Verification items for the finished model (mm, model axes). Face numbers are marked on the shaded views. Round coordinates to 2 decimals unless told otherwise and drop trailing zeros. Write each loop counter-clockwise with the first axis right and the second up, starting at its lowest first coordinate (ties: lowest second). Pieces come first, ordered by that corner, then holes. Notation, with made-up numbers: (-12, 28) - (23, 28) arc R16 ccw to (23, 38) - close; hole circle Ø10 at (61.25, 42). An arc over 180 degrees is marked (long way). Answer as a JSON object with one key per item and string values.
```python
from build123d import *

# Parameters (mm, degrees)
SKETCH1_R           = 25.5
SKETCH1_R_2         = 8.5
BOSS_EXTRUDE1_DEPTH = 5
CIRPATTERN1_COUNT   = 6


with BuildPart() as part:
    # Sketch1 → Boss-Extrude1 (new body)
    with BuildSketch(Plane.XY):
        Circle(SKETCH1_R)
        Circle(SKETCH1_R_2, mode=Mode.SUBTRACT)
    extrude(amount=BOSS_EXTRUDE1_DEPTH)

    # Sketch3 → M3 Clearance Hole1 (revolve, cut)
    with BuildSketch(Plane(origin=(0, 22.5, 5), x_dir=(0, -1, 0), z_dir=(1, 0, 0))):
        Polygon((0, 0), (0, 11.021463052), (1.7, 10), (1.7, 0), align=None)
    m3_clearance_hole1 = revolve(axis=Axis((0, 22.5, 11.35), (0, 0, -1)), mode=Mode.SUBTRACT)

    # Sketch5 → CSK for M3 Countersunk Flat Head Screw3 (revolve, cut)
    with BuildSketch(Plane(origin=(0, 11.5, 5), x_dir=(0, -1, 0), z_dir=(1, 0, 0))):
        Polygon((0, 0), (0, 11.021463052), (1.7, 10), (1.7, 1.45), (3.15, 0), align=None)
    csk_for_m3_countersunk_flat_head_screw3 = revolve(axis=Axis((0, 11.5, 11.35), (0, 0, -1)), mode=Mode.SUBTRACT)

    # CirPattern1: M3 Clearance Hole1, CSK for M3 Countersunk Flat Head Screw3 ×6 about axis
    cirpattern1_axis = Axis((0, 0, 0), (0, 0, 1))
    for i in range(1, CIRPATTERN1_COUNT):
        add(m3_clearance_hole1.rotate(cirpattern1_axis, i * 360 / CIRPATTERN1_COUNT), mode=Mode.SUBTRACT)
        add(csk_for_m3_countersunk_flat_head_screw3.rotate(cirpattern1_axis, i * 360 / CIRPATTERN1_COUNT), mode=Mode.SUBTRACT)


solid = part.part
```
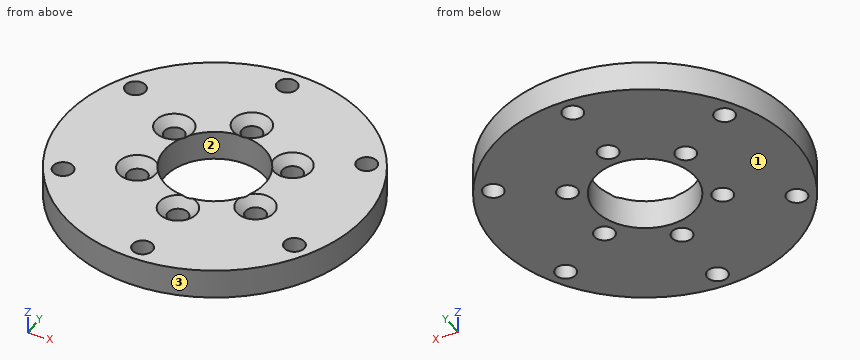
Q1. Material ranges on line 1 along Y through (x, z) = (0, 2.45); line 2 along X through (y, z) = (-7, 1.05); line 3 along Y through (x, z) = (20.5, 4.3), recorded low to high. Write a range as [from, to].
Geometry check:
{"line 1": "y = [-25.5, -24.2], [-20.8, -13.2], [-9.8, -8.5], [8.5, 9.8], [13.2, 20.8], [24.2, 25.5]", "line 2": "x = [-24.52, -11.11], [-8.81, -4.82], [4.82, 8.81], [11.11, 24.52]", "line 3": "y = [-15.17, -12.61], [-9.89, 9.89], [12.61, 15.17]"}
Q2. Gauge pin test, flat ends, axial feed: P1, Ø3, axis at x = -9.96, y = 5.75, coming from the +Z side; P2, Ø1.5, axis at x = -18.5, z = 2, coming from the +Y side; P3, Ø4, axis at x = -9.96, y = -5.75, coming from the +Z side; P4, Ø1, axis at x = 5, z = 2, coming from the -Y side. Record the tip position at first contact, or that the pin passes through.
Geometry check:
{"P1": "passes through", "P2": "stops at y = 18.31", "P3": "stops at z = 3.85", "P4": "stops at y = -25.1"}
Q3. Section check D-D, the plane y = -11.5. Record the cut outline in (x, z).
Geometry check:
{"outline": "(-22.76, 0) - (-21.17, 0) - (-21.17, 5) - (-22.76, 5) - close; (-17.8, 0) - (-1.7, 0) - (-1.7, 3.55) - (-3.15, 5) - (-17.8, 5) - close; (1.7, 0) - (17.8, 0) - (17.8, 5) - (3.15, 5) - (1.7, 3.55) - close; (21.17, 0) - (22.76, 0) - (22.76, 5) - (21.17, 5) - close"}
Q4. Section check C-C, the plane z = 0.9. State how many separate pieces and enclosed holes the cut face has, then the cut area to 3 significant figures.
Geometry check:
{"separate pieces": "1", "enclosed holes": "13", "area": "1,710 mm2"}
Q5. Section check A-A, the plane y = 22.5. Record the cut outline in (x, z).
Geometry check:
{"outline": "(-12, 0) - (-1.7, 0) - (-1.7, 5) - (-12, 5) - close; (1.7, 0) - (12, 0) - (12, 5) - (1.7, 5) - close"}
Q6. Release check for a two-part mould opening along Y. For the marked faces 1, 2 and 3 record: released by +Y, released by -Y, zero draft, split by the parting line, or undercut.
Geometry check:
{"face 1": "zero draft", "face 2": "undercut", "face 3": "split by the parting line"}
Q7. Section check B-B, the plane x = 0. Record the cut outline in (y, z), then the cut area to 3 significant figures.
Geometry check:
{"outline": "(-25.5, 0) - (-24.2, 0) - (-24.2, 5) - (-25.5, 5) - close; (-20.8, 0) - (-13.2, 0) - (-13.2, 3.55) - (-14.65, 5) - (-20.8, 5) - close; (-9.8, 0) - (-8.5, 0) - (-8.5, 4.85) - (-9.8, 3.55) - close; (8.5, 0) - (9.8, 0) - (9.8, 3.55) - (8.5, 4.85) - close; (13.2, 0) - (20.8, 0) - (20.8, 5) - (14.65, 5) - (13.2, 3.55) - close; (24.2, 0) - (25.5, 0) - (25.5, 5) - (24.2, 5) - close", "area": "97.8 mm2"}
